The figure shows three views and two pictorial views of one solid part (mm, origin at its lowest corner). Answer the questions. A direction names the side the tool comes from. Give positions to 0.01 mm unless a question says otherwise; leave off trailing zeros. Loops run counter-clockwise (first coordinate to the right, second up) from the corner with the lowest first, then second, coordinate; pieces in that order, holes last. Notation, with made-up numbers: M 62.5,-26.75 L 106.5,-26.75 A15 cw 106.5,0.25 Z; hole C -29.75,60 d4. An arc over 180 degrees is marked long. Write item = value, one per line. Start each with the question number.
1. Consider L1, parallel to Y at x = 150, z = 142.75; L2, parallel to Z at x = 200.5, y = 120; L3, parallel to Y at x = 151.5, z = 103 (1 decimal). Determine where each line is inside the solid, lowest interval first. Write a range as [from, to].
2. Section A-A on x = 150 is taken. Determine the outline of the cut face in (y, z).
3. Section B-B on y = 150 is taken. Determine the outline of the cut face in (x, z), plus the area to 3 significant figures.
4. The mould has two halves that part along Z. Classify the marked faces 1, 2 and 3: released by +Z, released by -Z, zero draft, split by the parting line, or undercut.
5. Section D-D on x = 55 is taken. Determine the outline of the cut face in (y, z), plus the area to 3 significant figures.
6. For the marked faces 4, 5, 6 and 7, determine the directions among +Z, -Z, +X, -X, +Y, -Y from which every point of the face is accessible in a straight line to the end or side of a thin tool.
7. Section C-C on y = 234 is taken. Determine the outline of the cut face in (x, z).
8. Flat-ended cylindrical pins translate along their axes: pin 1 Ø3 at (x, y) = (110, 238) entering from -Z; pin 2 Ø6 at (y, z) = (140.5, 6) entering from -X; pin 3 Ø10 at (x, z) = (150.5, 11) entering from +Y. Find the tip coordinate at first contact, or state that the pin passes through.
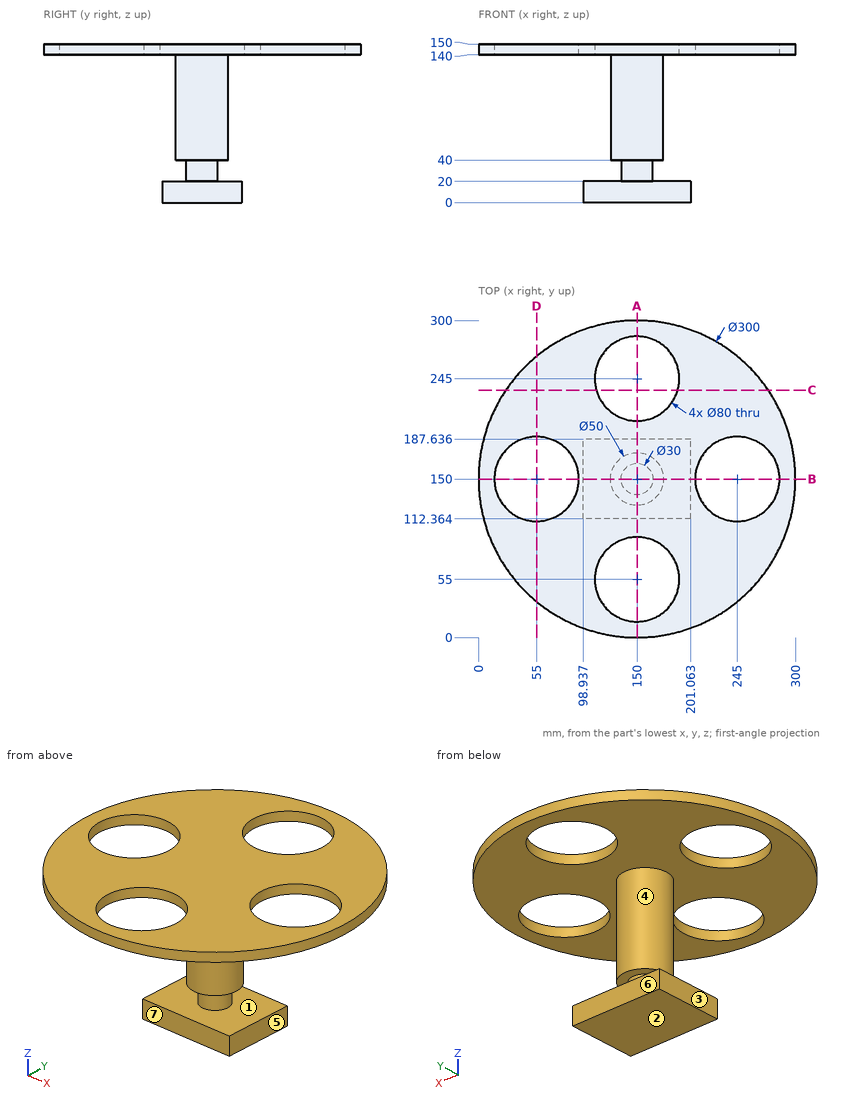
Verdict:
q1.L1 = [0, 15], [95, 205], [285, 300]
q1.L2 = [0, 20], [140, 150]
q1.L3 = [125, 175]
q2.outline = M 0,140 L 15,140 L 15,150 L 0,150 Z; M 95,140 L 125,140 L 125,40 L 135,40 L 135,20 L 112.36,20 L 112.36,0 L 187.64,0 L 187.64,20 L 165,20 L 165,40 L 175,40 L 175,140 L 205,140 L 205,150 L 95,150 Z; M 285,140 L 300,140 L 300,150 L 285,150 Z
q3.outline = M 0,140 L 15,140 L 15,150 L 0,150 Z; M 95,140 L 125,140 L 125,40 L 135,40 L 135,20 L 98.94,20 L 98.94,0 L 201.06,0 L 201.06,20 L 165,20 L 165,40 L 175,40 L 175,140 L 205,140 L 205,150 L 95,150 Z; M 285,140 L 300,140 L 300,150 L 285,150 Z
q3.area = 9,040 mm2
q4.face_1 = undercut
q4.face_2 = released by -Z
q4.face_3 = zero draft
q5.outline = M 33.92,140 L 110,140 L 110,150 L 33.92,150 Z; M 190,140 L 266.08,140 L 266.08,150 L 190,150 Z
q5.area = 1,520 mm2
q6.face_4 = none
q6.face_5 = -Z, +X, +Y, -Y
q6.face_6 = -Z, +X, -X, +Y
q6.face_7 = -Z, +X, -X, -Y
q7.outline = M 25.73,140 L 111.54,140 L 111.54,150 L 25.73,150 Z; M 188.46,140 L 274.27,140 L 274.27,150 L 188.46,150 Z
q8.pin_1 = 140
q8.pin_2 = 98.94
q8.pin_3 = 187.64
